For this review, take the finished solid that the model builds, in its own axes (mm). Face numbers are marked on the shaded views. Coordinates: 2 decimals unless noted, no trailing zeros. Loops run counter-clockwise (first coordinate to the right, second up) from the corner with the lowest first, then second, coordinate; pieces in that order, holes last. Notation, with made-up numbers: (0, 49) -> (52, 49) arc R17 cw to (52, 53) -> close; hole circle Ø4 at (41.5, 39.5). An arc over 180 degrees is marked (long way). Answer in a Markdown table with one row per item.
from build123d import *

# Parameters (mm, degrees)
F0_R      = 12
F1_DEPTH  = 2
F2_R      = 12
F2_R_2    = 4.5
F3_DEPTH  = 15
F4_R      = 12
F4_R_2    = 7.4
F5_DEPTH  = 107
F7_DEPTH  = 107.001
F8_R      = 1.5
F9_DEPTH  = 100
F10_R     = 12
F11_DEPTH = 10
F13_DEPTH = 10


with BuildPart() as f1:
    # F0 (on Top) → F1 (new body)
    with BuildSketch(Plane.XY):
        Circle(F0_R)
    extrude(amount=F1_DEPTH)

    # F2 (on face) → F3 (join)
    with BuildSketch(Plane.XY.offset(2)):
        Circle(F2_R)
        Circle(F2_R_2, mode=Mode.SUBTRACT)
    extrude(amount=F3_DEPTH)

    # F4 (on face) → F5 (join)
    with BuildSketch(Plane.XY.offset(17)):
        Circle(F4_R)
        Circle(F4_R_2, mode=Mode.SUBTRACT)
    extrude(amount=F5_DEPTH)

    # F6 (on face) → F7 (cut, through all)
    with BuildSketch(Plane.XY.offset(17)):
        Polygon((3.5, 0), (0, 0), (-3.5, 0), (-3.5, -10.5), (3.5, -10.5), align=None)
    extrude(amount=F7_DEPTH, mode=Mode.SUBTRACT)

    # F8 (on face) → F9 (cut)
    with BuildSketch(Plane.XY.offset(124)):
        with Locations((0, 9.5)):
            Circle(F8_R)
    extrude(amount=-F9_DEPTH, mode=Mode.SUBTRACT)

    # F10 (on face) → F11 (cut)
    with BuildSketch(Plane.XY.offset(124)):
        Circle(F10_R)
        with BuildLine():
            ThreePointArc((1.488384, 9.686316), (7.437276, 6.381765), (9.8, 0))
            ThreePointArc((9.8, 0), (8.072794, -5.556078), (3.5, -9.153688))
            Line((3.5, -9.153688), (3.5, -10.5))
            Line((3.5, -10.5), (-3.5, -10.5))
            Line((-3.5, -10.5), (-3.5, -9.153688))
            ThreePointArc((-3.5, -9.153688), (-9.74461, 1.040468), (-1.488384, 9.686316))
            ThreePointArc((-1.488384, 9.686316), (0, 11), (1.488384, 9.686316))
        make_face(mode=Mode.SUBTRACT)
    extrude(amount=-F11_DEPTH, mode=Mode.SUBTRACT)

    # F12 (on face) → F13 (cut)
    with BuildSketch(Plane.XY.offset(124)):
        Polygon((3.5, 0), (0, 0), (-3.5, 0), (-3.5, -12), (3.5, -12), align=None)
    extrude(amount=-F13_DEPTH, mode=Mode.SUBTRACT)


solid = f1.part
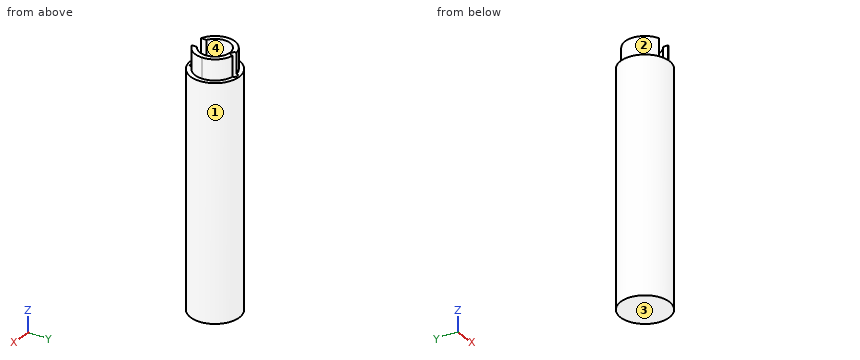
Item 1: Take a section at B-B, the plane z = 92. State the section outline as (x, y) points.
Worked answers:
| item | result |
|---|---|
| outline | circle Ø24 at (0, 0); hole (-3.5, -10.5) -> (3.5, -10.5) -> (3.5, -6.52) arc R7.4 ccw (long way) to (-3.5, -6.52) -> close; hole circle Ø3 at (0, 9.5) |
Item 2: Insertion check: pin 1 (12 mm diameter, centred on x = 0, y = 6, fed in from +Z); pin 2 (5 mm diameter, centred on y = 7, z = 91, fed in from +X); pin 3 (1.5 mm diameter, centred on x = 0.5, y = 9, fed in from +Z); pin 4 (1 mm diameter, centred on y = -2.5, z = 32, fed in from -X). Each pin has a flat end and moves straight along its axis. Give the tip position at first contact, or say it passes through.
Worked answers:
| item | result |
|---|---|
| pin 1 | z = 124 |
| pin 2 | x = 11.12 |
| pin 3 | z = 24 |
| pin 4 | x = -11.83 |
Item 3: The part is to be moulded in two halves that separate along X. For the marked faces 1, 2, 3 and 4, say which applies: +X half, -X half, draft (parallel to the pull), parting line (faces both ways), or undercut.
Worked answers:
| item | result |
|---|---|
| face 1 | parting line |
| face 2 | -X half |
| face 3 | draft |
| face 4 | undercut |
Item 4: Take a section at A-A, the plane x = 0. State the section outline as (y, z) points.
Worked answers:
| item | result |
|---|---|
| outline | (-12, 0) -> (12, 0) -> (12, 114) -> (11, 114) -> (11, 24) -> (8, 24) -> (8, 124) -> (7.4, 124) -> (7.4, 17) -> (4.5, 17) -> (4.5, 2) -> (-4.5, 2) -> (-4.5, 17) -> (-10.5, 17) -> (-10.5, 114) -> (-12, 114) -> close |
Item 5: For L1, parallel to Y at x = 0, z = 49.5; L2, parallel to X at y = -0.25, z = 42.5; L3, parallel to Y at x = 0.5, z = 51.5, list the stretches that pass through material, from the lowest coordinate up.
Worked answers:
| item | result |
|---|---|
| L1 | -12 to -10.5, 7.4 to 8, 11 to 12 |
| L2 | -12 to -7.4, 7.4 to 12 |
| L3 | -11.99 to -10.5, 7.38 to 8.09, 10.91 to 11.99 |
Item 6: Take a section at C-C, the plane x = -6. State the section outline as (y, z) points, and give its area (3 significant figures).
Worked answers:
| item | result |
|---|---|
| outline | (-10.39, 0) -> (10.39, 0) -> (10.39, 114) -> (7.75, 114) -> (7.75, 124) -> (4.33, 124) -> (4.33, 17) -> (-4.33, 17) -> (-4.33, 124) -> (-7.75, 124) -> (-7.75, 114) -> (-10.39, 114) -> close |
| area | 1,600 mm² |
